```python
from build123d import *

# Parameters (mm, degrees)
F1_W     = 100
F1_H     = 75
F1_W_2   = 90
F1_H_2   = 65
F2_DEPTH = 5
F3_DEPTH = 50
F5_DEPTH = 5


with BuildPart() as f2:
    # F1 (on face) → F2 (new body)
    with BuildSketch(Plane.XY):
        with Locations((1.0527614504, 8.5603988189)):
            Rectangle(F1_W, F1_H)
        with Locations((1.0527614504, 8.5603988189)):
            Rectangle(F1_W_2, F1_H_2, mode=Mode.SUBTRACT)
        with Locations((1.0527614504, 8.5603988189)):
            Rectangle(F1_W_2, F1_H_2)
    extrude(amount=F2_DEPTH)

    # F1 (on face) → F3 (join)
    with BuildSketch(Plane.XY):
        with Locations((1.0527614504, 8.5603988189)):
            Rectangle(F1_W, F1_H)
        with Locations((1.0527614504, 8.5603988189)):
            Rectangle(F1_W_2, F1_H_2, mode=Mode.SUBTRACT)
    extrude(amount=F3_DEPTH)

    # F4 (on face) → F5 (cut)
    with BuildSketch(Plane(origin=(0, 46.0603988189, 0), x_dir=(-1, 0, 0), z_dir=(0, 1, 0))):
        Polygon((-17.4, 45), (-22.5, 45), (-22.5, 40), (-22.5, 35), (-17.4, 35), (-17.4, 40), align=None)
        Polygon((2.55, 45), (-2.55, 45), (-2.55, 40), (-2.55, 35), (2.55, 35), (2.55, 40), align=None)
        Polygon((22.5, 45), (17.4, 45), (17.4, 40), (17.4, 35), (22.5, 35), align=None)
    extrude(amount=-F5_DEPTH, mode=Mode.SUBTRACT)


solid = f2.part
```
For this review, take the finished solid that the model builds, in its own axes (mm). A direction names the side the tool comes from. Round coordinates to 2 decimals unless told otherwise and drop trailing zeros. Write each loop counter-clockwise with the first axis right and the second up, starting at its lowest first coordinate (ties: lowest second). Pieces come first, ordered by that corner, then holes. Notation, with made-up numbers: (59.5, 88) -> (82.5, 88) arc R31 cw to (82.5, 117) -> close; hole circle Ø9 at (72, 78.25). An arc over 180 degrees is marked (long way). One line per question, with ' | ' between items. Start each with the question number.
1) Wall thickness on line 1 along X through (y, z) = (-22.5, 34); line 2 along Y through (x, z) = (20, 9); line 3 along Z through (x, y) = (-43, 18): over which ranges is each line inside the solid? List them lowest first.
2) Mouldability with a two-part tool opening along Y and no side actions: class faces 4 (the flat face through (0, -28.94, 25)), 5 (the flat face through (0, 9, 0)), 6 (the flat face through (46.053, 8, 27)) as +Y half, -Y half, draft (parallel to the pull), parting line (faces both ways), or undercut.
3) Add section C-C (x = -31). Write out the cut boundary in (y, z).
4) Add section B-B (y = -21). Write out the cut boundary in (x, z), and give its area (3 significant figures).
5) For pin 1 Ø1.5 at (x, y) = (-24, -4) entering from +Z, flat-tipped, find the tip position at first contact; note if it passes through.
6) Machinability: for faces 1 (the flat face through (20, 44, 45)), 2 (the flat face through (0, -23.94, 27)), 3 (the flat face through (51.053, 8, 25)), which of the approach directions +Z, -Z, +X, -X, +Y, -Y give a long, thin tool a straight path to every point of the face, cutting with its end or side? Answer none if there is none.
7) Add section A-A (z = 21.5). Write out the cut boundary in (x, y).
Reported:
1) line 1: x = -48.95 to -43.95, 46.05 to 51.05 | line 2: y = -28.94 to -23.94, 41.06 to 46.06 | line 3: z = 0 to 5
2) face 4: -Y half | face 5: draft | face 6: undercut
3) outline: (-28.94, 0) -> (46.06, 0) -> (46.06, 50) -> (41.06, 50) -> (41.06, 5) -> (-23.94, 5) -> (-23.94, 50) -> (-28.94, 50) -> close
4) outline: (-48.95, 0) -> (51.05, 0) -> (51.05, 50) -> (46.05, 50) -> (46.05, 5) -> (-43.95, 5) -> (-43.95, 50) -> (-48.95, 50) -> close | area: 950 mm²
5) pin 1: stops at z = 5
6) face 1: +Y | face 2: +Z | face 3: +Z, -Z, +X, +Y, -Y
7) outline: (-48.95, -28.94) -> (51.05, -28.94) -> (51.05, 46.06) -> (-48.95, 46.06) -> close; hole (-43.95, -23.94) -> (46.05, -23.94) -> (46.05, 41.06) -> (-43.95, 41.06) -> close
